The listing builds one solid part. Answer for the finished solid, in the listing's coordinates (mm). Face numbers are marked on the shaded views. A direction names the side the tool comes from. Round coordinates to 2 decimals unless told otherwise and drop trailing zeros. Write each loop counter-clockwise with the first axis right and the second up, starting at its lowest first coordinate (ties: lowest second). Pieces come first, ordered by that corner, then holes.
from build123d import *

# Parameters (mm, degrees)
SKETCH1_R             = 6
BOSS_EXTRUDE1_DEPTH   = 20
SKETCH2_R             = 5.25
BOSS_EXTRUDE2_DEPTH   = 20
CUT_EXTRUDE1_START    = -12
CUT_EXTRUDE1_DEPTH    = 12
M5_TAPPED_HOLE1_D     = 4.2
M5_TAPPED_HOLE1_DEPTH = 14
M5_TAPPED_HOLE1_TIP   = 1.2618073
SKETCH6_R             = 1.5
CUT_EXTRUDE2_DEPTH    = 42.72604103


with BuildPart() as part:
    # Sketch1 → Boss-Extrude1 (new body)
    with BuildSketch(Plane(origin=(0, 0, 0), x_dir=(1, 0, 0), z_dir=(0, 1, 0))):
        with Locations(Location((0, 0, 0), (0, 0, 270))):
            Circle(SKETCH1_R)
    extrude(amount=BOSS_EXTRUDE1_DEPTH)

    # Sketch2 → Boss-Extrude2 (add)
    with BuildSketch(Plane(origin=(0, 20, 0), x_dir=(1, 0, 0), z_dir=(0, 1, 0))):
        with Locations(Location((0, 0, 0), (0, 0, 270))):
            Circle(SKETCH2_R)
    extrude(amount=BOSS_EXTRUDE2_DEPTH)

    # Sketch3 → Cut-Extrude1 (cut)
    with BuildSketch(Plane(origin=(0, 40, 0), x_dir=(1, 0, 0), z_dir=(0, 1, 0)).offset(CUT_EXTRUDE1_START)):
        with BuildLine():
            Line((-3.082207001, 4.25), (3.082207001, 4.25))
            ThreePointArc((3.082207001, 4.25), (0, 5.25), (-3.082207001, 4.25))
        make_face()
    extrude(amount=CUT_EXTRUDE1_DEPTH, mode=Mode.SUBTRACT)

    # M5 Tapped Hole1
    with Locations(Plane(origin=(0, 40, 0), x_dir=(1, 0, 0), z_dir=(0, 1, 0))):
        with Locations((0, 0)):
            Hole(M5_TAPPED_HOLE1_D / 2, depth=M5_TAPPED_HOLE1_DEPTH)
            with Locations((0, 0, -(M5_TAPPED_HOLE1_DEPTH + M5_TAPPED_HOLE1_TIP / 2))):  # 118° drill point
                Cone(0, M5_TAPPED_HOLE1_D / 2, M5_TAPPED_HOLE1_TIP, mode=Mode.SUBTRACT)

    # Sketch6 → Cut-Extrude2 (cut, through all)
    with BuildSketch(Plane(origin=(0, 0, -4.25), x_dir=(-1, 0, 0), z_dir=(0, 0, -1))):
        with Locations((0, 37)):
            Circle(SKETCH6_R)
    extrude(amount=-CUT_EXTRUDE2_DEPTH, mode=Mode.SUBTRACT)

    # Chamfer1
    # the kernel refuses this chamfer: 1 mm, written as the material it adds along each edge
    with BuildSketch(Plane(origin=(0, 20, 0), x_dir=(0, 0, 1), z_dir=(-1, 0, 0))) as chamfer1_piece_1_section:
        with BuildLine():
            Line((6.278284271, -0.028284271), (5.221715729, 1.028284271))
            Line((5.221715729, 1.028284271), (5.201715729, 1.028284271))
            ThreePointArc((5.201715729, 1.028284271), (5.23, 0.514142136), (5.23, 0))
            Line((5.23, 0), (5.25, -0.02))
            ThreePointArc((5.25, -0.02), (5.764142136, -0.02), (6.278284271, -0.048284271))
            Line((6.278284271, -0.048284271), (6.278284271, -0.028284271))
        make_face()
    chamfer1_piece_1 = revolve(axis=Axis((0, 20, 0), (0, 1, 0)), mode=Mode.PRIVATE)
    chamfer1_piece_1 = chamfer1_piece_1 & Plane(origin=(0, 20.620713895, 0), x_dir=(0, 0, 1), z_dir=(0, -1, 0)) * Cylinder(6, 26, mode=Mode.PRIVATE)
    add(chamfer1_piece_1)
    # the kernel refuses this chamfer: 1 mm, written as the material it takes off along each edge
    with BuildSketch(Plane(origin=(0, 40, 0), x_dir=(0.522159484326456, 0, -0.8528478603642795), z_dir=(0.8528478603642795, 0, 0.522159484326456))) as chamfer1_2_piece_1:
        with BuildLine():
            Line((5.278284271, -1.028284271), (4.221715729, 0.028284271))
            Line((4.221715729, 0.028284271), (4.221715729, 0.048284271))
            ThreePointArc((4.221715729, 0.048284271), (4.735857864, 0.02), (5.25, 0.02))
            Line((5.25, 0.02), (5.27, 0))
            ThreePointArc((5.27, 0), (5.27, -0.514142136), (5.298284271, -1.028284271))
            Line((5.298284271, -1.028284271), (5.278284271, -1.028284271))
        make_face()
    revolve(axis=Axis((0, 40, 0), (0, 1, 0)), revolution_arc=211.477217225, mode=Mode.SUBTRACT)
    with BuildSketch(Plane(origin=(0, 40, 0), x_dir=(0, 0, 1), z_dir=(-1, 0, 0))) as chamfer1_2_piece_2:
        with BuildLine():
            Line((5.278284271, -1.028284271), (4.221715729, 0.028284271))
            Line((4.221715729, 0.028284271), (4.221715729, 0.048284271))
            ThreePointArc((4.221715729, 0.048284271), (4.735857864, 0.02), (5.25, 0.02))
            Line((5.25, 0.02), (5.27, 0))
            ThreePointArc((5.27, 0), (5.27, -0.514142136), (5.298284271, -1.028284271))
            Line((5.298284271, -1.028284271), (5.278284271, -1.028284271))
        make_face()
    revolve(axis=Axis((0, 40, 0), (0, 1, 0)), revolution_arc=211.477217225, mode=Mode.SUBTRACT)


solid = part.part
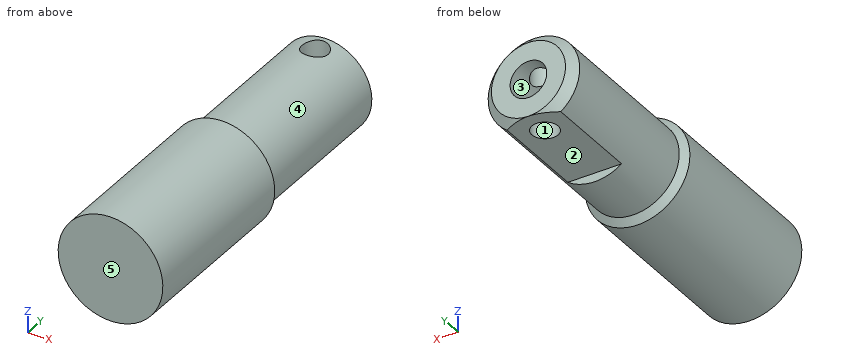
1. Given pin 1 (3 mm diameter, centred on y = 20.5, z = -3, fed in from +X); pin 2 (0.8 mm diameter, centred on x = 0, z = -5, fed in from +Y); pin 3 (4 mm diameter, centred on x = -2.5, y = 19.5, fed in from -Z), each flat-ended and moving along its own axis, determine where each tip first touches the part or whether it passes through.
Geometry says:
pin 1: stops at x = 5.8
pin 2: stops at y = 28
pin 3: stops at z = -5.98
2. Section B-B on x = 0.75 is taken. Give the number of separate pieces and of enclosed holes in the cut face, plus the area to 3 significant figures.
Geometry says:
separate pieces: 3
enclosed holes: 0
area: 364 mm2
3. A tool of negligible diameter and unlimited length cuts with its end or side. For the marked faces 1 and 2, from which of +Z, -Z, +X, -X, +Y, -Y can it reach the whole face along a straight path? Write none if from no direction.
Geometry says:
face 1: +Z, -Z
face 2: -Z, +X, -X, +Y
4. Section C-C on y = 27 is taken. Determine the outline of the cut face in (x, z).
Geometry says:
outline: circle Ø10.5 at (0, 0); hole circle Ø4.2 at (0, 0)
5. For a pull along Z with two mould halves and no side action, classify the marked faces 3, 4 and 5 as released by +Z, released by -Z, zero draft, split by the parting line, or undercut.
Geometry says:
face 3: undercut
face 4: split by the parting line
face 5: zero draft
6. Section D-D on y = 3.5 is taken. Determine the outline of the cut face in (x, z).
Geometry says:
outline: circle Ø12 at (0, 0)
7. Straight lines are drawn through the part: line 1 along Z through (x, y) = (0, 30.5); line 2 along Y through (x, z) = (0, 3.1); line 3 along X through (y, z) = (37, -2.8). For each, find the intervals that lie inside material, in ascending order.
Geometry says:
line 1: z = -4.25 to -2.1, 2.1 to 5.25
line 2: y = 0 to 35.5, 38.5 to 40
line 3: x = -4.44 to -1.5, 1.5 to 4.44
8. Section A-A on y = 37 is taken. Determine the outline of the cut face in (x, z), plus the area to 3 significant figures.
Geometry says:
outline: (-3.08, -4.25) - (-1.5, -4.25) - (-1.5, -1.47) arc R2.1 cw to (-1.5, 1.47) - (-1.5, 5.03) arc R5.25 ccw to start; (1.5, -4.25) - (3.08, -4.25) arc R5.25 ccw to (1.5, 5.03) - (1.5, 1.47) arc R2.1 cw to (1.5, -1.47) - close
area: 51.7 mm2
